Source: CAD feature listing. Evaluate the final solid. Frame: model axes, mm. A direction names the side the tool comes from. Give positions to 0.01 mm unless a question says otherwise; leave off trailing zeros. Write each loop counter-clockwise with the first axis right and the second up, starting at its lowest first coordinate (ties: lowest second). Pieces come first, ordered by that corner, then holes. Notation, with made-up numbers: (75, -6.75) -> (115, -6.75) arc R17 ccw to (115, 6.25) -> close; hole circle Ø1 at (-25.5, 22). An arc over 180 degrees is marked (long way). Write item = value, one per line.
from build123d import *

# Parameters (mm, degrees)
BOSS_EXTRUDE1_DEPTH = 9.525
FILLET1_R           = 3.175
BOSS_EXTRUDE2_DEPTH = 1.5875
SKETCH3_R           = 1.5875
CUT_EXTRUDE1_DEPTH  = 3.175
CHAMFER1_SIZE       = 1.5875
FILLET2_R           = 1.5875
FILLET3_R           = 3.9624


with BuildPart() as part:
    # Sketch1 → Boss-Extrude1 (new body, symmetric)
    with BuildSketch(Plane.XY):
        Polygon((-0.3175, -0.3175), (-0.3175, 25.7175), (1.3335, 25.7175), (1.3335, 22.225), (4.191, 22.225), (4.191, 28.575), (1.016, 28.575), (-3.175, 28.575), (-3.175, 1.5875), (-12.7, 1.5875), (-12.7, -1.5875), (-3.175, -1.5875), (4.191, -1.5875), (4.191, 0), (4.191, 3.175), (1.3335, 3.175), (1.3335, -0.3175), align=None)
    extrude(amount=BOSS_EXTRUDE1_DEPTH, both=True)

    # Fillet1
    fillet1_edges = [part.edges().sort_by_distance(p)[0] for p in [
        (-3.175, 1.5875, 0),
    ]]
    fillet(fillet1_edges, radius=FILLET1_R)

    # Sketch2 → Boss-Extrude2 (add, symmetric)
    with BuildSketch(Plane.XY):
        Polygon((-3.175, 28.575), (-12.7, 1.5875), (-3.175, 1.5875), align=None)
    extrude(amount=BOSS_EXTRUDE2_DEPTH, both=True)

    # Sketch3 → Cut-Extrude1 (cut)
    with BuildSketch(Plane(origin=(0, 1.5875, 0), x_dir=(1, 0, 0), z_dir=(0, 1, 0))):
        with Locations((-8.73125, -5.55625)):
            Circle(SKETCH3_R)
        with Locations((-8.73125, 5.55625)):
            Circle(SKETCH3_R)
    extrude(amount=-CUT_EXTRUDE1_DEPTH, mode=Mode.SUBTRACT)

    # Chamfer1
    chamfer1_edges = [part.edges().sort_by_distance(p)[0] for p in [
        (4.191, 3.175, 0),
        (4.191, 22.225, 0),
    ]]
    chamfer(chamfer1_edges, length=CHAMFER1_SIZE)

    # Fillet2
    fillet2_edges = [part.edges().sort_by_distance(p)[0] for p in [
        (0.508, 28.575, -9.525),
        (0.508, 28.575, 9.525),
    ]]
    fillet(fillet2_edges, radius=FILLET2_R)

    # Fillet3
    fillet3_edges = [part.edges().sort_by_distance(p)[0] for p in [
        (-12.7, 0, -9.525),
        (-12.7, 0, 9.525),
    ]]
    fillet(fillet3_edges, radius=FILLET3_R)


solid = part.part
1) Contact query for flat-ended pins moving along their axis: pin 1 (5 mm diameter, centred on x = -8.73, z = 5.56, fed in from +Y); pin 2 (2 mm diameter, centred on x = -11, y = 5.5, fed in from +Z); pin 3 (3 mm diameter, centred on y = 14.5, z = 6, fed in from +X); pin 4 (1 mm diameter, centred on y = 2, z = -3, fed in from -X). Output: stop coordinate, or through.
Computed:
pin_1 = 1.59
pin_2 = 1.59
pin_3 = -0.32
pin_4 = -12.7
2) Draft query along Y for faces 5 (the cylindrical face through (-4.13, 2.49, 5.61)), 6 (the flat face through (1.334, 24, 0)), 7 (the flat face through (1, -0.318, 0)), 8 (the cylindrical face through (-10, 0, -4.6)). Return one class per face: pulls with the +Y half, pulls with the -Y half, needs draft (parallel to the pull), parting line crosses it, or undercut.
Computed:
face_5 = pulls with the +Y half
face_6 = undercut
face_7 = undercut
face_8 = needs draft
3) Cut plane A-A (x = 0.75). Return the cut outline in (y, z) (1 decimal).
Computed:
outline = (-1.6, -9.5) -> (-0.3, -9.5) -> (-0.3, 9.5) -> (-1.6, 9.5) -> close; (25.7, -9.5) -> (27, -9.5) arc R1.6 ccw to (28.6, -7.9) -> (28.6, 7.9) arc R1.6 ccw to (27, 9.5) -> (25.7, 9.5) -> close
4) Material intervals for L1, parallel to Y at x = 2, z = -2.25 (1 decimal); L2, parallel to X at y = 6, z = 3.25 (1 decimal); L3, parallel to Y at x = -8.25, z = -2.5, sorted ascending.
Computed:
L1 = -1.6 to 3.2, 22.2 to 28.6
L2 = -3.2 to -0.3
L3 = -1.59 to 1.59
5) Cut plane D-D (y = 18). Return the cut outline in (x, z) (1 decimal), then the cut area to 3 significant figures.
Computed:
outline = (-6.9, -1.6) -> (-3.2, -1.6) -> (-3.2, -9.5) -> (-0.3, -9.5) -> (-0.3, 9.5) -> (-3.2, 9.5) -> (-3.2, 1.6) -> (-6.9, 1.6) -> close
area = 66.3 mm²
6) Access query for faces 1 (the flat face through (2, 22.225, 0)), 2 (the flat face through (-6, 9, -1.588)), 3 (the flat face through (-7.87, 15.27, 0.02)), 4 (the flat face through (0, 25.718, 0)). Directions: +Z, -Z, +X, -X, +Y, -Y. A direction counts if a zero-diameter tool reaches every point of the face in a straight line with its end or side. Return the directions, or none.
Computed:
face_1 = +Z, -Z, +X
face_2 = -Z, -X, +Y
face_3 = +Z, -Z, -X, +Y
face_4 = +Z, -Z
